```python
from build123d import *

# Parameters (mm, degrees)
PAD_DEPTH       = 3
SKETCH001_W     = 8
SKETCH001_H     = 3
PAD001_DEPTH    = 6.3
SKETCH002_W     = 8
SKETCH002_H     = 3
SKETCH002_W_2   = 21
PAD002_DEPTH    = 3
SKETCH003_R     = 3
POCKET_DEPTH    = 20
CHAMFER_SIZE2   = 4
CHAMFER_SIZE    = 4
FILLET001_R     = 5
FILLET002_R     = 1
POCKET001_DEPTH = 10
FILLET_R        = 2


with BuildPart() as part:
    # Sketch → Pad (new body)
    with BuildSketch(Plane.XY):
        Polygon((20, -10), (20, 10), (20, 13), (-20, 13), (-20, 10), (-20, -10), (-20, -13), (20, -13), align=None)
    extrude(amount=PAD_DEPTH)

    # Sketch001 (on Face4 of Pad) → Pad001 (join)
    with BuildSketch(Plane.XY.offset(3)):
        with Locations((16, 11.5)):
            Rectangle(SKETCH001_W, SKETCH001_H)
        with Locations((16, -11.5)):
            Rectangle(SKETCH001_W, SKETCH001_H)
        Polygon((11, 1.5), (11, 4.5), (1, 4.5), (1, 13), (-20, 13), (-20, -13), (1, -13), (1, -4.5), (11, -4.5), (11, -1.5), (5, -1.5), (5, 1.5), align=None)
    extrude(amount=PAD001_DEPTH)

    # Sketch002 (on Face5 of Pad001) → Pad002 (join)
    with BuildSketch(Plane.XY.offset(9.3)):
        with Locations((16, 11.5)):
            Rectangle(SKETCH002_W, SKETCH002_H)
        with Locations((-9.5, 11.5)):
            Rectangle(SKETCH002_W_2, SKETCH002_H)
        with Locations((16, -11.5)):
            Rectangle(SKETCH002_W, SKETCH002_H)
        with Locations((-9.5, -11.5)):
            Rectangle(SKETCH002_W_2, SKETCH002_H)
    extrude(amount=PAD002_DEPTH)

    # Sketch003 (on Face1 of Pad002) → Pocket (cut)
    with BuildSketch(Plane(origin=(0, 0, 0), x_dir=(1, 0, 0), z_dir=(0, 0, -1))):
        Circle(SKETCH003_R)
    extrude(amount=-POCKET_DEPTH, mode=Mode.SUBTRACT)

    # Chamfer
    chamfer_edges = [part.edges().sort_by_distance(p)[0] for p in [
        (-3, 0, 0),
    ]]
    chamfer_side = part.faces().sort_by_distance((-19.522926, 0, 0))[0]
    chamfer(chamfer_edges, length=CHAMFER_SIZE, length2=CHAMFER_SIZE2, reference=chamfer_side)

    # Fillet001
    fillet001_edges = [part.edges().sort_by_distance(p)[0] for p in [
        (1, 4.5, 6.15),
        (1, -4.5, 6.15),
    ]]
    fillet(fillet001_edges, radius=FILLET001_R)

    # Fillet002
    fillet002_edges = [part.edges().sort_by_distance(p)[0] for p in [
        (11, 4.5, 6.15),
        (12, 10, 7.65),
        (11, -4.5, 6.15),
        (12, -10, 7.65),
        (1, 13, 7.65),
        (12, 13, 7.65),
        (1, -13, 7.65),
        (12, -13, 7.65),
    ]]
    fillet(fillet002_edges, radius=FILLET002_R)

    # Fillet002 Face10 → Pocket001 (cut)
    with BuildSketch(Plane(origin=(-20, 0, 5.076097), x_dir=(0, 1, 0), z_dir=(-1, 0, 0))):
        Polygon((13, 5.076097), (-13, 5.076097), (-13, -7.223903), (-10, -7.223903), (-10, -4.223903), (10, -4.223903), (10, -7.223903), (13, -7.223903), align=None)
    extrude(amount=-POCKET001_DEPTH, mode=Mode.SUBTRACT)

    # Fillet
    fillet_edges = [part.edges().sort_by_distance(p)[0] for p in [
        (-10, 13, 6.15),
        (20, 13, 6.15),
        (20, -13, 6.15),
        (-10, -13, 6.15),
    ]]
    fillet(fillet_edges, radius=FILLET_R)


solid = part.part
```
Can you work these out from the model? Positions are in its coordinate system, mm. A direction names the side the tool comes from. Give positions to 0.01 mm unless a question says otherwise; leave off trailing zeros. Order: outer loops, then holes, each group sorted by start corner. A loop starts at its lowest first (then second) coordinate and runs counter-clockwise, first axis right, second up. Notation, with made-up numbers: M 88.5,72 L 100.5,72 A13 cw 100.5,96 Z; hole C -37,-14.5 d2. An arc over 180 degrees is marked long. One line per item, written item: value.
1) Please list where these lines run through material, in increasing order: line 1 along X through (y, z) = (0, 5.4); line 2 along X through (y, z) = (-3.5, 6); line 3 along Z through (x, y) = (7, -7).
Answer sheet:
line 1: x = -10 to -3, 3 to 5
line 2: x = -10 to 11
line 3: z = 0 to 3
2) I want a section at B-B, the plane x = -7.5. List the corners of the cut face in (y, z) for me.
Answer sheet:
outline: M -13,0 L 13,0 L 13,12.3 L 10,12.3 L 10,9.3 L -10,9.3 L -10,12.3 L -13,12.3 Z
3) I want a section at A-A, the plane y = 0. List the corners of the cut face in (x, z) for me, plus the area to 3 significant figures.
Answer sheet:
outline: M -10,0 L -7,0 L -3,4 L -3,9.3 L -10,9.3 Z; M 3,4 L 7,0 L 20,0 L 20,3 L 5,3 L 5,9.3 L 3,9.3 Z
area: 113 mm^2
4) I want a section at C-C, the plane z = 1.5. List the corners of the cut face in (x, y) for me, plus the area to 3 significant figures.
Answer sheet:
outline: M -10,-11 A2 ccw -8,-13 L 18,-13 A2 ccw 20,-11 L 20,11 A2 ccw 18,13 L -8,13 A2 ccw -10,11 Z; hole C 0,0 d11
area: 682 mm^2
5) For P1, Ø5, axis at y = -5, z = 7.5, coming from the +X side; P2, Ø3, axis at x = 14, y = 5, coming from the +Z side; P3, Ø1.8, axis at x = 8.5, z = 5.5, coming from the -Y side; P4, Ø5, axis at x = 8.5, z = 3.5, coming from the +Y side, each with a flat end and sliding along its axis, tell me the tip position at first contact or that it passes through.
Answer sheet:
P1: stops at x = 11
P2: stops at z = 3
P3: stops at y = -4.5
P4: stops at y = 13
6) I want a section at D-D, the plane x = 15. List the corners of the cut face in (y, z) for me.
Answer sheet:
outline: M -13,0 L 13,0 L 13,12.3 L 10,12.3 L 10,3 L -10,3 L -10,12.3 L -13,12.3 Z
7) On a 3-axis mill with a long thin cutter (end or side, diameter ignored), from which of +Z, -Z, +X, -X, +Y, -Y can I reach the whole of each face in a straight line? I mean faces 4 (the face through (5, 0, 6)), 5 (the face through (-5, -10, 11)), 6 (the face through (1, 11, 8)). Say none if no direction works.
Answer sheet:
face 4: +Z, +X
face 5: +Z, +X, -X
face 6: +Z, +Y
8) We'd pull the mould along X, two halves only. Please class faces 1 (the face through (16, -11, 12.3)), 2 (the face through (11, -3, 6)), 3 (the face through (12.301, -12.715, 7.715)): released by +X, released by -X, zero draft, split by the parting line, or undercut.
Answer sheet:
face 1: zero draft
face 2: released by +X
face 3: undercut
